Geometry: final body of the model. Coordinates: model frame, mm. A direction names the side the tool comes from. Round coordinates to 2 decimals unless told otherwise and drop trailing zeros. Order: outer loops, then holes, each group sorted by start corner. A loop starts at its lowest first (then second) coordinate and runs counter-clockwise, first axis right, second up. Notation, with made-up numbers: (-19.75, 75) - (-13.75, 75) arc R11 cw to (-13.75, 93) - close; hole circle Ø8 at (-19, 81). An arc over 180 degrees is marked (long way). Put each result on its own line as item: value. Start each with the question number.
(1) Section B-B (z = 0). Output: boundary loops of the cut face in (x, y), and give its area (3 significant figures).
(2) Pin query (flat end, axial travel): P1, Ø3.5, axis at x = 48.5, y = 29, coming from the +Z side; P2, Ø12, axis at y = 44, z = 0, coming from the +X side; P3, Ø0.7, axis at x = -40, z = 21, coming from the -Y side; P4, Ø9.5, axis at x = 48, y = 43, coming from the -Z side. Return the tip coordinate at first contact, or that it passes through.
(3) Material intervals for L1, parallel to Y at x = -48, z = 0; L2, parallel to Z at x = -37.62, y = 3.3; L3, parallel to X at y = 1.05, z = 0, sorted ascending. Write a range as [from, to].
(4) Section D-D (x = 0). Output: boundary loops of the cut face in (y, z).
(5) Section C-C (x = -37.62). Output: boundary loops of the cut face in (y, z).
(6) Pull-direction query (Y, two-part tool) for faces 1 (the face through (11, 0, -1)), 2 (the face through (-45.92, 34.24, -2.17)), 3 (the face through (46, 35, 40)); classes: released by +Y, released by -Y, zero draft, split by the parting line, or undercut.
(7) Section A-A (y = 19). Output: boundary loops of the cut face in (x, z).
(8) Access query for faces 4 (the face through (40, 28, 1)), 5 (the face through (-35.09, 2.46, 23.33)), 6 (the face through (-46, 35, -40)). Directions: +Z, -Z, +X, -X, +Y, -Y. A direction counts if a zero-diameter tool reaches every point of the face in a straight line with its end or side. Return the directions, or none.
from build123d import *

# Parameters (mm, degrees)
SKETCH1_W               = 104
SKETCH1_H               = 100
SKETCH1_R               = 3
SKETCH1_R_2             = 6
BOSS_EXTRUDE1_DEPTH     = 5
SKETCH2_W               = 12
SKETCH2_H               = 80
BOSS_EXTRUDE2_DEPTH     = 60
CUT_EXTRUDE1_DEPTH      = 133.442440328
CUT_EXTRUDE1_DEPTH_BACK = 133.442440328
SKETCH3_R               = 10


with BuildPart() as part:
    # Sketch1 → Boss-Extrude1 (new body)
    with BuildSketch(Plane(origin=(0, 0, 0), x_dir=(1, 0, 0), z_dir=(0, 1, 0))):
        Rectangle(SKETCH1_W, SKETCH1_H)
        with Locations(Location((-37.62, -21.72, 0), (0, 0, 270))):
            Circle(SKETCH1_R, mode=Mode.SUBTRACT)
        with Locations(Location((37.62, -21.72, 0), (0, 0, 90))):
            Circle(SKETCH1_R, mode=Mode.SUBTRACT)
        with Locations(Location((37.62, 21.72, 0), (0, 0, 270))):
            Circle(SKETCH1_R, mode=Mode.SUBTRACT)
        with Locations(Location((-37.62, 21.72, 0), (0, 0, 90))):
            Circle(SKETCH1_R, mode=Mode.SUBTRACT)
        with Locations(Location((0, 0, 0), (0, 0, 270))):
            Circle(SKETCH1_R_2, mode=Mode.SUBTRACT)
    extrude(amount=BOSS_EXTRUDE1_DEPTH)

    # Sketch2 → Boss-Extrude2 (add)
    with BuildSketch(Plane(origin=(0, 5, 0), x_dir=(1, 0, 0), z_dir=(0, 1, 0))):
        with Locations((-46, 0)):
            Rectangle(SKETCH2_W, SKETCH2_H)
        with Locations((46, 0)):
            Rectangle(SKETCH2_W, SKETCH2_H)
    extrude(amount=BOSS_EXTRUDE2_DEPTH)

    # Sketch3 → Cut-Extrude1 (cut, two sides: drawn at the far end of the back side and taken through both)
    with BuildSketch(Plane.ZY.offset(52).offset(-CUT_EXTRUDE1_DEPTH_BACK)):
        with Locations((0, 44)):
            Circle(SKETCH3_R)
    extrude(amount=CUT_EXTRUDE1_DEPTH + CUT_EXTRUDE1_DEPTH_BACK, mode=Mode.SUBTRACT)


solid = part.part
Checks:
1. outline: (-52, 0) - (-6, 0) - (-6, 5) - (-40, 5) - (-40, 34) - (-52, 34) - close; (-52, 54) - (-40, 54) - (-40, 65) - (-52, 65) - close; (6, 0) - (52, 0) - (52, 34) - (40, 34) - (40, 5) - (6, 5) - close; (40, 54) - (52, 54) - (52, 65) - (40, 65) - close
1. area: 1,420 mm²
2. P1: stops at z = 40
2. P2: passes through
2. P3: stops at y = 5
2. P4: stops at z = -40
3. L1: y = [0, 34], [54, 65]
3. L2: z = [-50, -24.72], [-18.72, 18.72], [24.72, 50]
3. L3: x = [-52, -6], [6, 52]
4. outline: (0, -50) - (5, -50) - (5, -6) - (0, -6) - close; (0, 6) - (5, 6) - (5, 50) - (0, 50) - close
5. outline: (0, -50) - (5, -50) - (5, -24.72) - (0, -24.72) - close; (0, -18.72) - (5, -18.72) - (5, 18.72) - (0, 18.72) - close; (0, 24.72) - (5, 24.72) - (5, 50) - (0, 50) - close
6. face 1: released by -Y
6. face 2: undercut
6. face 3: zero draft
7. outline: (-52, -40) - (-40, -40) - (-40, 40) - (-52, 40) - close; (40, -40) - (52, -40) - (52, 40) - (40, 40) - close
8. face 4: +Z, -Z, +Y
8. face 5: -Y
8. face 6: -Z, +X, -X, +Y
